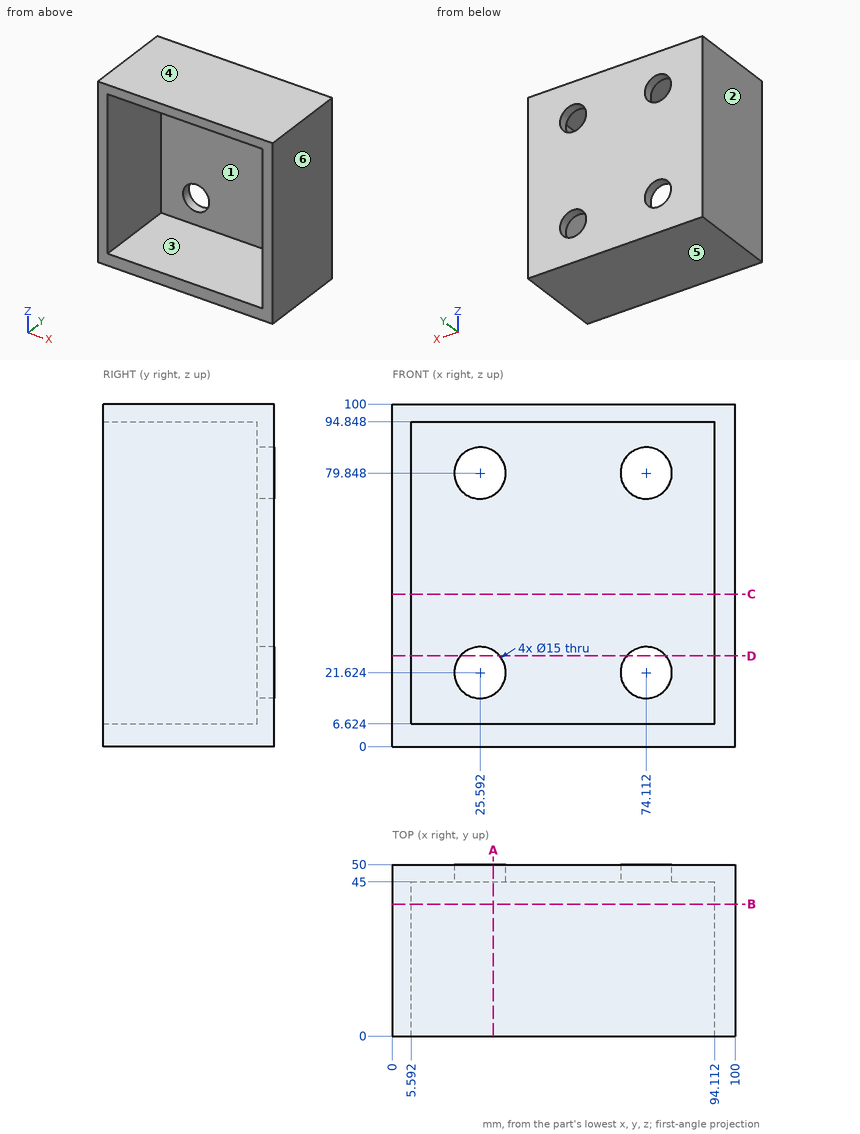
Geometry: see drawing. Coordinates: mm, zero at the bounding-box minimum. A direction names the side the tool comes from. Give positions to 0.01 mm unless a question says otherwise; leave off trailing zeros. Loops run counter-clockwise (first coordinate to the right, second up) from the corner with the lowest first, then second, coordinate; pieces in that order, holes last. Notation, with made-up numbers: M 21,70 L 44,70 A23 ccw 44,79 Z; hole C 76.25,-15.5 d6. An arc over 180 degrees is marked long. Use one line per item in the form item = value.
1. First-contact query: pin 1 (13.5 mm diameter, centred on x = 25.59, z = 21.62, fed in from -Y); pin 2 (2 mm diameter, centred on x = 61.5, z = 63.5, fed in from -Y). Flat tips, straight axial feed; report the tip coordinate or a pass-through.
Numbers:
pin_1 = through
pin_2 = 45
2. Pull-direction query (Z, two-part tool) for the marked faces 3, 4, 5 and 6; classes: released by +Z, released by -Z, zero draft, split by the parting line, or undercut.
Numbers:
face_3 = undercut
face_4 = released by +Z
face_5 = released by -Z
face_6 = zero draft
3. Line query: L1, parallel to Z at x = 25, y = 20 (1 decimal); L2, parallel to X at y = 21, z = 65; L3, parallel to Y at x = 78, z = 28.5. Output: solid intervals per line, ascending.
Numbers:
L1 = 0 to 6.6, 94.8 to 100
L2 = 0 to 5.59, 94.11 to 100
L3 = 45 to 50
4. Section query D-D, the plane z = 26.5. Return the cut outline in (x, y).
Numbers:
outline = M 0,0 L 5.59,0 L 5.59,45 L 19.89,45 L 19.89,50 L 0,50 Z; M 31.29,45 L 68.41,45 L 68.41,50 L 31.29,50 Z; M 79.81,45 L 94.11,45 L 94.11,0 L 100,0 L 100,50 L 79.81,50 Z
5. Section query C-C, the plane z = 44.5. Return the cut outline in (x, y), and give its area (3 significant figures).
Numbers:
outline = M 0,0 L 5.59,0 L 5.59,45 L 94.11,45 L 94.11,0 L 100,0 L 100,50 L 0,50 Z
area = 1,020 mm²
6. Section query A-A, the plane x = 29.5. Count the separate pieces of the cut face and the enclosed holes in it, and give its area (3 significant figures).
Numbers:
separate_pieces = 3
enclosed_holes = 0
area = 902 mm²
7. Reachability of the marked faces 1 and 2 from +Z, -Z, +X, -X, +Y, -Y: full face, straight path, thin tool, end or side. Return the list, or none.
Numbers:
face_1 = -Y
face_2 = +Z, -Z, -X, +Y, -Y
8. Section query B-B, the plane y = 38.5. Return the cut outline in (x, z) (1 decimal), and give its area (3 significant figures).
Numbers:
outline = M 0,0 L 100,0 L 100,100 L 0,100 Z; hole M 5.6,6.6 L 94.1,6.6 L 94.1,94.8 L 5.6,94.8 Z
area = 2,190 mm²
